from build123d import *

# Parameters (mm, degrees)
SKETCH1_R               = 6.75
BOSS_EXTRUDE1_DEPTH     = 9
SKETCH2_R               = 5
BOSS_EXTRUDE2_DEPTH     = 1
CUT_EXTRUDE1_DEPTH      = 14.119641763
CUT_EXTRUDE1_DEPTH_BACK = 14.119641763
SKETCH3_W               = 1.75
SKETCH3_H               = 7.4
CUT_EXTRUDE2_DEPTH      = 14.119641763
CUT_EXTRUDE2_DEPTH_BACK = 14.119641763
SKETCH4_W               = 7.4
SKETCH4_H               = 4.85
SKETCH4_H_2             = 2.35
CUT_EXTRUDE3_DEPTH      = 17.267298485
CUT_EXTRUDE3_DEPTH_BACK = 17.267298485
SKETCH5_R               = 1
CHAMFER1_SIZE           = 2


with BuildPart() as part:
    # Sketch1 → Boss-Extrude1 (new body)
    with BuildSketch(Plane.XY):
        Circle(SKETCH1_R)
    extrude(amount=BOSS_EXTRUDE1_DEPTH)

    # Sketch2 → Boss-Extrude2 (add)
    with BuildSketch(Plane(origin=(0, 0, 0), x_dir=(-1, 0, 0), z_dir=(0, 0, -1))):
        Circle(SKETCH2_R)
    extrude(amount=BOSS_EXTRUDE2_DEPTH)

    # Sketch3 → Cut-Extrude1 (cut, two sides: drawn at the far end of the back side and taken through both)
    with BuildSketch(Plane(origin=(0, 0, 0), x_dir=(1, 0, 0), z_dir=(0, 1, 0)).offset(-CUT_EXTRUDE1_DEPTH_BACK)):
        with Locations((-5.875, -5.3)):
            Rectangle(SKETCH3_W, SKETCH3_H)
        with Locations((5.875, -5.3)):
            Rectangle(SKETCH3_W, SKETCH3_H)
    extrude(amount=CUT_EXTRUDE1_DEPTH + CUT_EXTRUDE1_DEPTH_BACK, mode=Mode.SUBTRACT)

    # Sketch4 → Cut-Extrude2 (cut, two sides: drawn at the far end of the back side and taken through both)
    with BuildSketch(Plane(origin=(0, 0, 0), x_dir=(0, 0, -1), z_dir=(1, 0, 0)).offset(-CUT_EXTRUDE2_DEPTH_BACK)):
        with Locations((-5.3, -4.325)):
            Rectangle(SKETCH4_W, SKETCH4_H)
        with Locations((-5.3, 5.575)):
            Rectangle(SKETCH4_W, SKETCH4_H_2)
    extrude(amount=CUT_EXTRUDE2_DEPTH + CUT_EXTRUDE2_DEPTH_BACK, mode=Mode.SUBTRACT)

    # Sketch5 → Cut-Extrude3 (cut, two sides: drawn at the far end of the back side and taken through both)
    with BuildSketch(Plane(origin=(5, 0, 0), x_dir=(0, 0, -1), z_dir=(1, 0, 0)).offset(-CUT_EXTRUDE3_DEPTH_BACK)):
        with Locations((-7, 0)):
            Circle(SKETCH5_R)
    extrude(amount=CUT_EXTRUDE3_DEPTH + CUT_EXTRUDE3_DEPTH_BACK, mode=Mode.SUBTRACT)

    # Chamfer1
    chamfer1_edges = [part.edges().sort_by_distance(p)[0] for p in [
        (0, -1.9, 9),
    ]]
    chamfer(chamfer1_edges, length=CHAMFER1_SIZE)


solid = part.part
Source: CAD feature listing. Evaluate the final solid. Frame: model axes, mm. A direction names the side the tool comes from. Round coordinates to 2 decimals unless told otherwise and drop trailing zeros. Loops run counter-clockwise (first coordinate to the right, second up) from the corner with the lowest first, then second, coordinate; pieces in that order, holes last. Notation, with made-up numbers: (20.5, 9) - (28.5, 9) arc R33 cw to (28.5, 45) - close; hole circle Ø8 at (28.5, 16). An arc over 180 degrees is marked (long way). Write item = value, one per line. Start each with the question number.
(1) Section query C-C, the plane z = 1. Output: boundary loops of the cut face in (x, y), plus the area to 3 significant figures.
(2) Pin query (flat end, axial travel): pin 1 (4.5 mm diameter, centred on x = 2, z = 5, fed in from -Y); pin 2 (6 mm diameter, centred on y = 5, z = 1, fed in from -X); pin 3 (5 mm diameter, centred on y = 4, z = 4.5, fed in from +X); pin 4 (6 mm diameter, centred on x = 0, z = 4, fed in from +Y). Return the tip coordinate at first contact, or that it passes through.
(3) Section query B-B, the plane z = 7.5. Output: boundary loops of the cut face in (x, y), plus the area to 3 significant figures.
(4) Ray query, line 1 along Z through (x, y) = (0.5, -3.25); line 2 along X through (y, z) = (-0.5, 4.5); line 3 along Z through (x, y) = (1.5, 0). Return the intervals inside material, ascending. Write a range as from..to.
(5) Section query D-D, the plane y = -5.25. Output: boundary loops of the cut face in (x, z).
(6) Set-up query: faces 1 (the face through (0, 4.4, 5)), 2 (the face through (-5, -2, 0)), 3 (the face through (0, -1.9, 4)). Return all of +Z, -Z, +X, -X, +Y, -Y with unobstructed straight access to the full face (end or side cutting, diameter ignored); none if empty.
(7) Pull-direction query (Z, two-part tool) for faces 4 (the face through (-0.1, -0.6, 7.8)), 5 (the face through (0, 0, -1)), 6 (the face through (0, 2, 9)); classes: +Z half, -Z half, draft (parallel to the pull), parting line (faces both ways), or undercut.
(8) Section query A-A, the plane x = 0. Output: boundary loops of the cut face in (y, z), plus the area to 3 significant figures.
Conclusion:
q1.outline = circle Ø13.5 at (0, 0)
q1.area = 143 mm2
q2.pin_1 = -1.9
q2.pin_2 = -6.45
q2.pin_3 = 5
q2.pin_4 = 6.75
q3.outline = (-5, -1.4) - (5, -1.4) - (5, -0.87) - (-5, -0.87) - close; (-5, 0.87) - (5, 0.87) - (5, 4.4) - (-5, 4.4) - close
q3.area = 40.7 mm2
q4.line_1 = -1..1.6
q4.line_2 = -5..5
q4.line_3 = -1..6, 8..8.9
q5.outline = (-4.24, 0) - (4.24, 0) - (4.24, 1.6) - (-4.24, 1.6) - close
q6.face_1 = +Z, +X, -X, +Y
q6.face_2 = -Z
q6.face_3 = +Z, +X, -X, -Y
q7.face_4 = undercut
q7.face_5 = -Z half
q7.face_6 = +Z half
q8.outline = (-6.75, 0) - (-5, 0) - (-5, -1) - (5, -1) - (5, 0) - (6.75, 0) - (6.75, 1.6) - (4.4, 1.6) - (4.4, 9) - (0.1, 9) - (-1.9, 7) - (-1.9, 1.6) - (-6.75, 1.6) - close; hole circle Ø2 at (0, 7)
q8.area = 73.1 mm2
